The model under review builds one solid part; all positions refer to its coordinate system, in mm. A direction names the side the tool comes from. Round coordinates to 2 decimals unless told otherwise and drop trailing zeros. Write each loop counter-clockwise with the first axis right and the second up, starting at its lowest first coordinate (ties: lowest second). Pieces come first, ordered by that corner, then holes.
Item 1: Draft analysis for pull direction Y (two halves, no side actions). For faces 1 (the face through (-3.521, 9.536, -0.325)), 2 (the face through (0, 1, 15)), 3 (the face through (5.6, 3.57, 0.07)), state which applies: +Y half, -Y half, draft (parallel to the pull), parting line (faces both ways), or undercut.
Item 2: Add section A-A (y = 15). Give the boundary of the cut face in (x, z), plus the area to 3 significant figures.
Item 3: Add section B-B (x = -13). Give the boundary of the cut face in (y, z).
Item 4: Add section D-D (x = -22). Give the boundary of the cut face in (y, z).
Item 5: Machinability: for faces 4 (the face through (-3, 7, 5)), 5 (the face through (2, 9, 0)), 6 (the face through (5, 9, 0)), which of the approach directions +Z, -Z, +X, -X, +Y, -Y give a long, thin tool a straight path to every point of the face, cutting with its end or side? Answer none if there is none.
Item 6: To check wall thickness, follow L1, parallel to X at y = 1.9, z = 0; L2, parallel to Y at x = -3.1, z = 0; L3, parallel to X at y = 14.5, z = -1.5. State the ranges of each line that lie inside material, in increasing order.
Item 7: Clearance check with flat-ended pins moving along their axes: pin 1 Ø6 at (x, z) = (-21.5, 3) entering from +Y; pin 2 Ø2.5 at (x, y) = (-4.5, 7) entering from +Z; pin 3 Ø5 at (x, z) = (-15, 0) entering from +Y; pin 4 Ø1.5 at (x, z) = (-7, -4.5) entering from +Y. State where each tip first meets the part, or that it passes through.
Item 8: Add section C-C (z = -3.5). Give the boundary of the cut face in (x, y).
```python
from build123d import *

# Parameters (mm, degrees)
CROQUIS1_W              = 60
CROQUIS1_H              = 30
SALIENTE_EXTRUIR1_DEPTH = 3
CROQUIS2_R              = 4.25
CORTAR_EXTRUIR1_DEPTH   = 3
REDONDEO1_R             = 5
CROQUIS4_W              = 3
CROQUIS4_H              = 10
SALIENTE_EXTRUIR2_DEPTH = 13
CORTAR_EXTRUIR2_DEPTH   = 13
CROQUIS6_R              = 1.5
CORTAR_EXTRUIR3_DEPTH   = 13
SALIENTE_EXTRUIR3_DEPTH = 10


with BuildPart() as part:
    # Croquis1 → Saliente-Extruir1 (new body)
    with BuildSketch(Plane(origin=(0, 0, 0), x_dir=(1, 0, 0), z_dir=(0, 1, 0))):
        Rectangle(CROQUIS1_W, CROQUIS1_H)
    extrude(amount=SALIENTE_EXTRUIR1_DEPTH)

    # Croquis2 → Cortar-Extruir1 (cut)
    with BuildSketch(Plane(origin=(0, 3, 0), x_dir=(1, 0, 0), z_dir=(0, 1, 0))):
        with Locations(Location((-15, 0, 0), (0, 0, 270))):
            Circle(CROQUIS2_R)
        with Locations(Location((15, 0, 0), (0, 0, 270))):
            Circle(CROQUIS2_R)
    extrude(amount=-CORTAR_EXTRUIR1_DEPTH, mode=Mode.SUBTRACT)

    # Redondeo1
    redondeo1_edges = [part.edges().sort_by_distance(p)[0] for p in [
        (30, 1.5, 15),
        (-30, 1.5, 15),
        (-30, 1.5, -15),
        (30, 1.5, -15),
    ]]
    fillet(redondeo1_edges, radius=REDONDEO1_R)

    # Croquis4 → Saliente-Extruir2 (add)
    with BuildSketch(Plane(origin=(0, 3, 0), x_dir=(1, 0, 0), z_dir=(0, 1, 0))):
        with Locations((-3.5, 0)):
            Rectangle(CROQUIS4_W, CROQUIS4_H)
        with Locations((3.5, 0)):
            Rectangle(CROQUIS4_W, CROQUIS4_H)
    extrude(amount=SALIENTE_EXTRUIR2_DEPTH)

    # Croquis5 → Cortar-Extruir2 (cut)
    with BuildSketch(Plane(origin=(5, 0, 0), x_dir=(0, 0, -1), z_dir=(1, 0, 0))):
        with BuildLine():
            Line((-5, 16), (-5, 11))
            ThreePointArc((-5, 11), (-3.535533906, 14.535533906), (0, 16))
            Line((0, 16), (-5, 16))
        make_face()
        with BuildLine():
            ThreePointArc((0, 16), (3.535533906, 14.535533906), (5, 11))
            Line((5, 11), (5, 16))
            Line((5, 16), (0, 16))
        make_face()
    extrude(amount=-CORTAR_EXTRUIR2_DEPTH, mode=Mode.SUBTRACT)

    # Croquis6 → Cortar-Extruir3 (cut)
    with BuildSketch(Plane.ZY.offset(5)):
        with Locations((0, 11)):
            Circle(CROQUIS6_R)
    extrude(amount=-CORTAR_EXTRUIR3_DEPTH, mode=Mode.SUBTRACT)

    # Croquis7 → Saliente-Extruir3 (add)
    with BuildSketch(Plane.XY.offset(5)):
        with BuildLine():
            Line((-7, 3), (-5, 3))
            Line((-5, 3), (-5, 5))
            ThreePointArc((-5, 5), (-5.585786438, 3.585786438), (-7, 3))
        make_face()
        with BuildLine():
            Line((5, 5), (5, 3))
            Line((5, 3), (7, 3))
            ThreePointArc((7, 3), (5.585786438, 3.585786438), (5, 5))
        make_face()
    extrude(amount=-SALIENTE_EXTRUIR3_DEPTH)


solid = part.part
```
Numbers:
1. face 1: undercut
1. face 2: draft
1. face 3: +Y half
2. outline: (-5, -3) - (-2, -3) - (-2, 3) - (-5, 3) - close; (2, -3) - (5, -3) - (5, 3) - (2, 3) - close
2. area: 36.0 mm2
3. outline: (0, -15) - (3, -15) - (3, -3.75) - (0, -3.75) - close; (0, 3.75) - (3, 3.75) - (3, 15) - (0, 15) - close
4. outline: (0, -15) - (3, -15) - (3, 15) - (0, 15) - close
5. face 4: +Z, +X, -X, +Y
5. face 5: +Z, -Z, +Y
5. face 6: +Z, -Z, +X, +Y
6. L1: x = -30 to -19.25, -10.75 to 10.75, 19.25 to 30
6. L2: y = 0 to 9.5, 12.5 to 16
6. L3: x = -5 to -2, 2 to 5
7. pin 1: stops at y = 3
7. pin 2: stops at z = 5
7. pin 3: passes through
7. pin 4: stops at y = 3.15
8. outline: (-30, 0) - (-17.41, 0) - (-17.41, 3) - (-30, 3) - close; (-12.59, 0) - (12.59, 0) - (12.59, 3) - (7, 3) arc R2 cw to (5, 5) - (5, 14.57) - (2, 14.57) - (2, 3) - (-2, 3) - (-2, 14.57) - (-5, 14.57) - (-5, 5) arc R2 cw to (-7, 3) - (-12.59, 3) - close; (17.41, 0) - (30, 0) - (30, 3) - (17.41, 3) - close
